The listing builds one solid part. Answer for the finished solid, in the listing's coordinates (mm). Face numbers are marked on the shaded views. Round coordinates to 2 decimals unless told otherwise and drop trailing zeros. Write each loop counter-clockwise with the first axis right and the second up, starting at its lowest first coordinate (ties: lowest second). Pieces come first, ordered by that corner, then holes.
(1) A cutting plane is placed at D-D, the plane z = -8.5. Give the vertices of the cut face in (x, y) (1 decimal).
(2) A cutting plane is placed at A-A, the plane x = 0. Give the vertices of the cut face in (y, z) (1 decimal), and give its area (3 significant figures).
(3) The mould has two halves that part along Y. Classify the marked faces 1, 2, 3 and 4: +Y half, -Y half, draft (parallel to the pull), parting line (faces both ways), or undercut.
(4) A cutting plane is placed at B-B, the plane z = -13.5. Give the vertices of the cut face in (x, y) (1 decimal).
(5) Each of these flat-tipped pins is pushed along its axis until it touches: pin 1 Ø1 at (x, z) = (-9, -5) entering from +Y; pin 2 Ø3 at (x, z) = (3.5, -17) entering from -Y; pin 3 Ø4 at (y, z) = (5, -18) entering from -X. Where does it stop, or does it pass through?
(6) A cutting plane is placed at C-C, the plane y = 5.25. Give the vertices of the cut face in (x, z) (3 decimals).
(7) Find the intervals of material crossed by probe 1 along Z at (x, y) = (0, -3.75) (3 decimals); probe 2 along X at (y, z) = (1.5, -6); probe 3 along X at (y, z) = (-6, -12.7), in increasing order.
from build123d import *

# Parameters (mm, degrees)
SKETCH2_R              = 11.1125
BOSS_EXTRUDE1_DEPTH    = 22.225
F_10_24_TAPPED_HOLE1_D = 3.7973
SKETCH7_W              = 1.89865
SKETCH7_H              = 11.1125
F_10_24_TAPPED_HOLE3_D = 3.7973


with BuildPart() as part:
    # Sketch2 → Boss-Extrude1 (new body)
    with BuildSketch(Plane.XY):
        Circle(SKETCH2_R)
    extrude(amount=-BOSS_EXTRUDE1_DEPTH)

    # #10-24 Tapped Hole1 (through all)
    with Locations(Plane.XY):
        with Locations((0, 0)):
            Hole(F_10_24_TAPPED_HOLE1_D / 2)

    # Sketch7 → #10-24 Tapped Hole2 (revolve, cut)
    with BuildSketch(Plane(origin=(0, 0, -12.7), x_dir=(0, 0, -1), z_dir=(1, 0, 0))):
        with Locations((0.949325, 5.55625)):
            Rectangle(SKETCH7_W, SKETCH7_H)
    revolve(axis=Axis((0, -6.35, -12.7), (0, 1, 0)), mode=Mode.SUBTRACT)

    # #10-24 Tapped Hole3 (through all)
    with Locations(Plane(origin=(0, 0, 0), x_dir=(1, 0, 0), z_dir=(0, 1, 0))):
        with Locations((0, 12.7)):
            Hole(F_10_24_TAPPED_HOLE3_D / 2)


solid = part.part
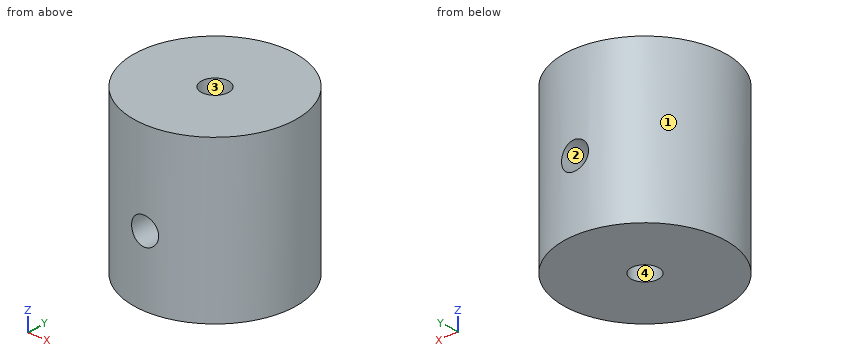
Solutions:
1. outline: circle Ø22.2 at (0, 0); hole circle Ø3.8 at (0, 0)
2. outline: (-11.1, -22.2) - (-1.9, -22.2) - (-1.9, -14.6) - (-11.1, -14.6) - close; (-11.1, -10.8) - (-1.9, -10.8) - (-1.9, 0) - (-11.1, 0) - close; (1.9, -22.2) - (11.1, -22.2) - (11.1, -14.6) - (1.9, -14.6) - close; (1.9, -10.8) - (11.1, -10.8) - (11.1, 0) - (1.9, 0) - close
2. area: 340 mm2
3. face 1: parting line
3. face 2: draft
3. face 3: undercut
3. face 4: undercut
4. outline: (-1.7, -11) - (-1.7, -0.8) arc R1.9 cw to (-1.7, 0.8) - (-1.7, 11) arc R11.1 ccw to start; (1.7, -11) arc R11.1 ccw to (1.7, 11) - (1.7, 0.8) arc R1.9 cw to (1.7, -0.8) - close
5. pin 1: stops at y = 7.16
5. pin 2: stops at y = -10.93
5. pin 3: stops at x = -10.7
6. outline: (-9.794, -22.225) - (9.794, -22.225) - (9.794, 0) - (-9.794, 0) - close; hole circle Ø3.797 at (0, -12.7)
7. probe 1: z = -22.225 to -14.599, -10.801 to 0
7. probe 2: x = -11.01 to -1.16, 1.16 to 11.01
7. probe 3: x = -9.35 to -1.9, 1.9 to 9.35
